Source: CAD feature listing. Evaluate the final solid. Frame: model axes, mm. A direction names the side the tool comes from. Give positions to 0.01 mm unless a question says otherwise; leave off trailing zeros. Order: outer loops, then holes, each group sorted by start corner. A loop starts at its lowest first (then second) coordinate and runs counter-clockwise, first axis right, second up.
from build123d import *

# Parameters (mm, degrees)
SKETCH1_R               = 1.5
BOSS_EXTRUDE1_DEPTH     = 28.5
SKETCH2_R               = 3
BOSS_EXTRUDE2_DEPTH     = 37
SKETCH5_R               = 5
BOSS_EXTRUDE3_DEPTH     = 1.8
SKETCH6_R               = 3
BOSS_EXTRUDE4_DEPTH     = 7.4
SKETCH3_W               = 2.2
SKETCH3_H               = 7.5
CUT_EXTRUDE1_DEPTH      = 6
CUT_EXTRUDE1_DEPTH_BACK = 6
SKETCH4_R               = 1
CUT_EXTRUDE2_DEPTH      = 6
CUT_EXTRUDE2_DEPTH_BACK = 6


with BuildPart() as part:
    # Sketch1 → Boss-Extrude1 (new body, symmetric)
    with BuildSketch(Plane.XY):
        Circle(SKETCH1_R)
    extrude(amount=BOSS_EXTRUDE1_DEPTH, both=True)

    # Sketch2 → Boss-Extrude2 (add)
    with BuildSketch(Plane.XY.offset(28.5)):
        Circle(SKETCH2_R)
    extrude(amount=-BOSS_EXTRUDE2_DEPTH)

    # Sketch5 → Boss-Extrude3 (add)
    with BuildSketch(Plane.XY.offset(18.5)):
        Circle(SKETCH5_R)
    extrude(amount=BOSS_EXTRUDE3_DEPTH)

    # Sketch6 → Boss-Extrude4 (add)
    with BuildSketch(Plane(origin=(0, 0, -21.1), x_dir=(-1, 0, 0), z_dir=(0, 0, -1))):
        Circle(SKETCH6_R)
    extrude(amount=BOSS_EXTRUDE4_DEPTH)

    # Sketch3 → Cut-Extrude1 (cut, two sides)
    with BuildSketch(Plane(origin=(0, 0, 0), x_dir=(1, 0, 0), z_dir=(0, 1, 0))) as cut_extrude1_sk:
        with Locations((0, -24.75)):
            Rectangle(SKETCH3_W, SKETCH3_H)
    extrude(amount=CUT_EXTRUDE1_DEPTH, mode=Mode.SUBTRACT)
    extrude(cut_extrude1_sk.sketch, amount=-CUT_EXTRUDE1_DEPTH_BACK, mode=Mode.SUBTRACT)

    # Sketch4 → Cut-Extrude2 (cut, two sides)
    with BuildSketch(Plane(origin=(0, 0, 0), x_dir=(0, 0, -1), z_dir=(1, 0, 0))) as cut_extrude2_sk:
        with Locations((-26, 0)):
            Circle(SKETCH4_R)
    extrude(amount=CUT_EXTRUDE2_DEPTH, mode=Mode.SUBTRACT)
    extrude(cut_extrude2_sk.sketch, amount=-CUT_EXTRUDE2_DEPTH_BACK, mode=Mode.SUBTRACT)


solid = part.part
1) Section query D-D on z = -13.5. Output: boundary loops of the cut face in (x, y).
Checks:
outline: circle Ø3 at (0, 0)
2) First-contact query: pin 1 Ø1.8 at (x, y) = (0.5, -1) entering from +Z; pin 2 Ø3 at (y, z) = (0, 26) entering from +X; pin 3 Ø2 at (x, y) = (-2, 3.5) entering from +Z; pin 4 Ø6 at (y, z) = (2.5, -16) entering from -X. Flat tips, straight axial feed; report the tip coordinate or a pass-through.
Checks:
pin 1: stops at z = 28.5
pin 2: stops at x = 3
pin 3: stops at z = 20.3
pin 4: stops at x = -1.5
3) Pull-direction query (X, two-part tool) for faces 1 (the face through (1.3, -1.3, -8.5)), 2 (the face through (-1.5, 0.07, -14.71)), 3 (the face through (1.1, 0, 24.8)); classes: +X half, -X half, draft (parallel to the pull), parting line (faces both ways), or undercut.
Checks:
face 1: draft
face 2: parting line
face 3: undercut
4) Ray query, L1, parallel to Z at x = 2.55, y = 0; L2, parallel to Z at x = 2, y = 1.5; L3, parallel to Z at x = -1.25, y = -4. Return the intervals inside material, ascending.
Checks:
L1: z = -28.5 to -21.1, -8.5 to 25, 27 to 28.5
L2: z = -28.5 to -21.1, -8.5 to 28.5
L3: z = 18.5 to 20.3
5) Reachability of faces 4 (the face through (2, 0, 28.5)), 5 (the face through (-1.3, -1.3, -21.1)), 6 (the face through (3, 0, -25)), 7 (the face through (-0.1, -3.3, 20.3)), 8 (the face through (0, 0, 21)) from +Z, -Z, +X, -X, +Y, -Y: full face, straight path, thin tool, end or side. Return the list, or none.
Checks:
face 4: +Z, +X, -X, +Y, -Y
face 5: none
face 6: -Z
face 7: +Z
face 8: +Z, +Y, -Y
6) Section query C-C on x = 0. Output: boundary loops of the cut face in (y, z).
Checks:
outline: (-5, 18.5) - (-3, 18.5) - (-3, -8.5) - (-1.5, -8.5) - (-1.5, -21.1) - (-3, -21.1) - (-3, -28.5) - (3, -28.5) - (3, -21.1) - (1.5, -21.1) - (1.5, -8.5) - (3, -8.5) - (3, 18.5) - (5, 18.5) - (5, 20.3) - (3, 20.3) - (3, 21) - (-3, 21) - (-3, 20.3) - (-5, 20.3) - close
7) Section query A-A on y = 0. State how many separate pieces and enclosed holes the cut face has, and give its area (3 significant figures).
Checks:
separate pieces: 3
enclosed holes: 0
area: 287 mm2
8) Section query B-B on z = 26. Output: boundary loops of the cut face in (x, y), and give its area (3 significant figures).
Checks:
outline: (-2.83, -1) arc R3 ccw to (-1.1, -2.79) - (-1.1, -1) - close; (-2.83, 1) - (-1.1, 1) - (-1.1, 2.79) arc R3 ccw to start; (1.1, -2.79) arc R3 ccw to (2.83, -1) - (1.1, -1) - close; (1.1, 1) - (2.83, 1) arc R3 ccw to (1.1, 2.79) - close
area: 8.00 mm2
